CAD build for the part. Positions are in the model's coordinates, mm. A direction names the side the tool comes from. Round coordinates to 2 decimals unless told otherwise and drop trailing zeros. Write each loop counter-clockwise with the first axis right and the second up, starting at its lowest first coordinate (ties: lowest second). Pieces come first, ordered by that corner, then holes. Notation, with made-up numbers: (21.25, -13) - (33.25, -13) arc R35 cw to (33.25, 22) - close; hole circle Ø6 at (30.5, 41). An arc over 180 degrees is marked (long way). Use one line per item in the form item = value. Start each with the question number.
Item 1: Band-saw the part on D-D, the plane z = -4. List the corners of the cut face in (x, y), and give its area (3 significant figures).
Item 2: Pin check, flat tips, straight feed: pin 1 (1.8 mm diameter, centred on x = -16, y = 0, fed in from -Z); pin 2 (5 mm diameter, centred on x = 20, y = 0, fed in from -Z); pin 3 (2 mm diameter, centred on x = -2.5, z = -1, fed in from +Y); pin 4 (3 mm diameter, centred on x = 0.5, y = 0.5, fed in from -Z). Stop position of each tip, or through.
Item 3: Tool access for faces 4 (the cylindrical face through (3, 0, -3)), 5 (the cylindrical face through (10.5, 0.07, 1.27)), 6 (the flat face through (1.3, -1.3, 1.5)): list every direction of +Z, -Z, +X, -X, +Y, -Y with a clear straight run to the whole face (end or side of a thin tool).
Item 4: Drill centre lines: L1, parallel to Z at x = 6.5, y = 1.75; L2, parallel to Y at x = 1, z = 1.25; L3, parallel to Z at x = -2, y = -0.5. Where is each one in solid material? Low to high.
Item 5: Band-saw the part on A-A, the plane z = 1. List the corners of the cut face in (x, y).
Item 6: Band-saw the part on C-C, the plane y = 0. Give the number of separate pieces and of enclosed holes in the cut face, and give its area (3 significant figures).
Item 7: Pull direction Y, two halves, no side cores. Call faces 1 (the flat face through (10, 0, 0)), 2 (the flat face through (11.091, 3.487, 1.232)), 3 (the flat face through (-1.3, -1.3, -1.6)): +Y half, -Y half, draft (parallel to the pull), parting line (faces both ways), or undercut.
Item 8: Band-saw the part on B-B, the plane x = -20. List the corners of the cut face in (y, z).
from build123d import *

# Parameters (mm, degrees)
EXTRUDE_2_DEPTH     = 2.5
CUT_EXTRUDE_1_REACH = 4.5
SKETCH_3_R          = 1.5
SKETCH_5_R          = 5
EXTRUDE_3_DEPTH     = 7.5
SKETCH_6_R          = 3
CUT_EXTRUDE_2_DEPTH = 3.4
SKETCH_7_R          = 1.5
CUT_EXTRUDE_3_DEPTH = 5.1
SKETCH_8_R          = 3
CUT_EXTRUDE_4_DEPTH = 1


with BuildPart() as part:
    # 草图1 → 凸台-拉伸2 (new body)
    with BuildSketch(Plane.XY):
        with BuildLine():
            Line((-21.779069767, 1.980434312), (-0.697674419, 4.95108578))
            ThreePointArc((-0.697674419, 4.95108578), (0, 5), (0.697674419, 4.95108578))
            Line((0.697674419, 4.95108578), (21.779069767, 1.980434312))
            ThreePointArc((21.779069767, 1.980434312), (23.5, 0), (21.779069767, -1.980434312))
            Line((21.779069767, -1.980434312), (0.697674419, -4.95108578))
            ThreePointArc((0.697674419, -4.95108578), (0, -5), (-0.697674419, -4.95108578))
            Line((-0.697674419, -4.95108578), (-21.779069767, -1.980434312))
            ThreePointArc((-21.779069767, -1.980434312), (-23.5, 0), (-21.779069767, 1.980434312))
        make_face()
    extrude(amount=EXTRUDE_2_DEPTH)

    # 草图3 → 切除-拉伸1 (cut, up to next)
    with BuildSketch(Plane.XY.offset(2.5), mode=Mode.PRIVATE) as cut_extrude_1_sk1:
        with Locations((-12, 0)):
            Circle(SKETCH_3_R)
    cut_extrude_1_tool1 = extrude(cut_extrude_1_sk1.sketch, amount=-CUT_EXTRUDE_1_REACH, mode=Mode.PRIVATE) & part.part
    add(cut_extrude_1_tool1.solids().sort_by_distance((-12, 0, 2.5))[0], mode=Mode.SUBTRACT)
    # 草图3 → 切除-拉伸1 (cut, up to next)
    with BuildSketch(Plane.XY.offset(2.5), mode=Mode.PRIVATE) as cut_extrude_1_sk2:
        with Locations((-16, 0)):
            Circle(SKETCH_3_R)
    cut_extrude_1_tool2 = extrude(cut_extrude_1_sk2.sketch, amount=-CUT_EXTRUDE_1_REACH, mode=Mode.PRIVATE) & part.part
    add(cut_extrude_1_tool2.solids().sort_by_distance((-16, 0, 2.5))[0], mode=Mode.SUBTRACT)
    # 草图3 → 切除-拉伸1 (cut, up to next)
    with BuildSketch(Plane.XY.offset(2.5), mode=Mode.PRIVATE) as cut_extrude_1_sk3:
        with Locations((-20, 0)):
            Circle(SKETCH_3_R)
    cut_extrude_1_tool3 = extrude(cut_extrude_1_sk3.sketch, amount=-CUT_EXTRUDE_1_REACH, mode=Mode.PRIVATE) & part.part
    add(cut_extrude_1_tool3.solids().sort_by_distance((-20, 0, 2.5))[0], mode=Mode.SUBTRACT)
    # 草图3 → 切除-拉伸1 (cut, up to next)
    with BuildSketch(Plane.XY.offset(2.5), mode=Mode.PRIVATE) as cut_extrude_1_sk4:
        with Locations((12, 0)):
            Circle(SKETCH_3_R)
    cut_extrude_1_tool4 = extrude(cut_extrude_1_sk4.sketch, amount=-CUT_EXTRUDE_1_REACH, mode=Mode.PRIVATE) & part.part
    add(cut_extrude_1_tool4.solids().sort_by_distance((12, 0, 2.5))[0], mode=Mode.SUBTRACT)
    # 草图3 → 切除-拉伸1 (cut, up to next)
    with BuildSketch(Plane.XY.offset(2.5), mode=Mode.PRIVATE) as cut_extrude_1_sk5:
        with Locations((16, 0)):
            Circle(SKETCH_3_R)
    cut_extrude_1_tool5 = extrude(cut_extrude_1_sk5.sketch, amount=-CUT_EXTRUDE_1_REACH, mode=Mode.PRIVATE) & part.part
    add(cut_extrude_1_tool5.solids().sort_by_distance((16, 0, 2.5))[0], mode=Mode.SUBTRACT)
    # 草图3 → 切除-拉伸1 (cut, up to next)
    with BuildSketch(Plane.XY.offset(2.5), mode=Mode.PRIVATE) as cut_extrude_1_sk6:
        with Locations((20, 0)):
            Circle(SKETCH_3_R)
    cut_extrude_1_tool6 = extrude(cut_extrude_1_sk6.sketch, amount=-CUT_EXTRUDE_1_REACH, mode=Mode.PRIVATE) & part.part
    add(cut_extrude_1_tool6.solids().sort_by_distance((20, 0, 2.5))[0], mode=Mode.SUBTRACT)

    # 草图5 → 凸台-拉伸3 (add)
    with BuildSketch(Plane.XY.offset(2.5)):
        Circle(SKETCH_5_R)
    extrude(amount=-EXTRUDE_3_DEPTH)

    # 草图6 → 切除-拉伸2 (cut)
    with BuildSketch(Plane(origin=(0, 0, -5), x_dir=(-1, 0, 0), z_dir=(0, 0, -1))):
        Circle(SKETCH_6_R)
    extrude(amount=-CUT_EXTRUDE_2_DEPTH, mode=Mode.SUBTRACT)

    # 草图7 → 切除-拉伸3 (cut, through all)
    with BuildSketch(Plane(origin=(0, 0, -1.6), x_dir=(-1, 0, 0), z_dir=(0, 0, -1))):
        Circle(SKETCH_7_R)
    extrude(amount=-CUT_EXTRUDE_3_DEPTH, mode=Mode.SUBTRACT)

    # 草图8 → 切除-拉伸4 (cut)
    with BuildSketch(Plane.XY.offset(2.5)):
        Circle(SKETCH_8_R)
    extrude(amount=-CUT_EXTRUDE_4_DEPTH, mode=Mode.SUBTRACT)


solid = part.part
Determined:
q1.outline = circle Ø10 at (0, 0); hole circle Ø6 at (0, 0)
q1.area = 50.3 mm²
q2.pin_1 = through
q2.pin_2 = 0
q2.pin_3 = 4.77
q2.pin_4 = -1.6
q3.face_4 = -Z
q3.face_5 = +Z, -Z
q3.face_6 = +Z
q4.L1 = 0 to 2.5
q4.L2 = -4.91 to -1.12, 1.12 to 4.91
q4.L3 = -1.6 to 1.5
q5.outline = (-21.78, -1.98) - (-0.7, -4.95) arc R5 ccw to (0.7, -4.95) - (21.78, -1.98) arc R2 ccw to (21.78, 1.98) - (0.7, 4.95) arc R5 ccw to (-0.7, 4.95) - (-21.78, 1.98) arc R2 ccw to start; hole circle Ø3 at (-20, 0); hole circle Ø3 at (-16, 0); hole circle Ø3 at (-12, 0); hole circle Ø3 at (0, 0); hole circle Ø3 at (12, 0); hole circle Ø3 at (16, 0); hole circle Ø3 at (20, 0)
q6.separate_pieces = 8
q6.enclosed_holes = 0
q6.area = 86.8 mm²
q7.face_1 = draft
q7.face_2 = +Y half
q7.face_3 = undercut
q8.outline = (-2.23, 0) - (-1.5, 0) - (-1.5, 2.5) - (-2.23, 2.5) - close; (1.5, 0) - (2.23, 0) - (2.23, 2.5) - (1.5, 2.5) - close
